Read the model definition and answer for the solid it produces. Units are mm, in the model's axes. Face numbers are marked on the shaded views. Give positions to 0.01 mm unless a question says otherwise; leave off trailing zeros. Write each loop counter-clockwise with the first axis right and the second up, starting at its lowest first coordinate (ties: lowest second). Pieces come first, ordered by that corner, then holes. Notation, with made-up numbers: M -16.5,-2 L -6.5,-2 A13 ccw -6.5,18 Z; hole C 5,-9 d1. An arc over 180 degrees is marked long. Write each question's results on one line, items separated by ' | '. Start each with the question number.
```python
from build123d import *

# Parameters (mm, degrees)
F0_R          = 76.2
F1_DEPTH      = 6.35
F3_R          = 38.1
F3_R_2        = 31.75
F4_DEPTH      = 6.35
F4_DEPTH_BACK = 6.35
F5_W          = 3.175
F5_H          = 3.175
F6_DEPTH      = 12.7


with BuildPart() as f1:
    # F0 (on Top) → F1 (new body)
    with BuildSketch(Plane.XY):
        Circle(F0_R)
        with BuildLine():
            Line((-41.613887, -47.963887), (-23.981943, -30.331943))
            Line((-23.981943, -30.331943), (-6.35, -63.181702))
            ThreePointArc((-6.35, -63.181702), (-25.160069, -58.302838), (-41.613887, -47.963887))
        make_face(mode=Mode.SUBTRACT)
        with BuildLine():
            ThreePointArc((-47.963887, -41.613887), (-58.302838, -25.160069), (-63.181702, -6.35))
            Line((-63.181702, -6.35), (-6.35, -6.35))
            Line((-6.35, -6.35), (-47.963887, -41.613887))
        make_face(mode=Mode.SUBTRACT)
        with BuildLine():
            Line((6.35, -63.181702), (6.35, -37.940851))
            Line((6.35, -37.940851), (41.613887, -47.963887))
            ThreePointArc((41.613887, -47.963887), (25.160069, -58.302838), (6.35, -63.181702))
        make_face(mode=Mode.SUBTRACT)
        with BuildLine():
            Line((47.963887, -41.613887), (6.35, -6.35))
            Line((6.35, -6.35), (63.181702, -6.35))
            ThreePointArc((63.181702, -6.35), (58.302838, -25.160069), (47.963887, -41.613887))
        make_face(mode=Mode.SUBTRACT)
        with BuildLine():
            Line((-6.35, 63.181702), (-5.498498, 19.546218))
            Line((-5.498498, 19.546218), (-8.109563, 21.600755))
            Line((-8.109563, 21.600755), (-6.35, 6.35))
            Line((-6.35, 6.35), (-63.181702, 6.35))
            ThreePointArc((-63.181702, 6.35), (-56.377813, 29.219723), (-41.613887, 47.963887))
            ThreePointArc((-41.613887, 47.963887), (-28.119246, 56.934682), (-12.793478, 62.197885))
            ThreePointArc((-12.793478, 62.197885), (-9.584371, 62.772525), (-6.35, 63.181702))
        make_face(mode=Mode.SUBTRACT)
        with BuildLine():
            Line((10.118387, 39.011938), (6.35, 37.940851))
            Line((6.35, 37.940851), (6.35, 63.181702))
            ThreePointArc((6.35, 63.181702), (9.584371, 62.772525), (12.793478, 62.197885))
            ThreePointArc((12.793478, 62.197885), (28.119246, 56.934682), (41.613887, 47.963887))
            ThreePointArc((41.613887, 47.963887), (56.377813, 29.219723), (63.181702, 6.35))
            Line((63.181702, 6.35), (6.35, 6.35))
            Line((6.35, 6.35), (10.118387, 39.011938))
        make_face(mode=Mode.SUBTRACT)
    extrude(amount=F1_DEPTH)

    # F3 (on offset) → F4 (join, two sides)
    with BuildSketch(Plane.XY.offset(3.175)) as f4_sk:
        Circle(F3_R)
        Circle(F3_R_2, mode=Mode.SUBTRACT)
    extrude(amount=F4_DEPTH)
    extrude(f4_sk.sketch, amount=-F4_DEPTH_BACK)

    # F5 (on Top) → F6 (cut, symmetric)
    with BuildSketch(Plane.XY):
        Rectangle(F5_W, F5_H)
    extrude(amount=F6_DEPTH, both=True, mode=Mode.SUBTRACT)


solid = f1.part
```
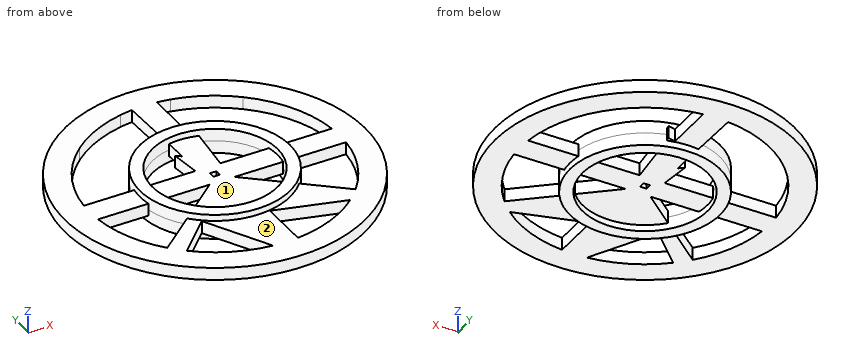
Item 1: Determine the mould class of the marked faces 1 and 2 for opening direction Y: +Y half, -Y half, draft (parallel to the pull), parting line (faces both ways), or undercut.
Item 2: Section B-B, the plane x = 55 is taken. Determine the outline of the cut face in (y, z).
Item 3: Section D-D, the plane y = -18 is taken. Give the number of separate pieces and of enclosed holes in the cut face, then the cut area to 3 significant figures.
Item 4: Straight lines are drawn through the part: line 1 (Y direction, x = 0, z = -0.5); line 2 (X direction, y = -49.5, z = 1.5); line 3 (X direction, y = -53, z = 4) (3 decimals). For each, find the intervals that lie inside material, in ascending order.
Item 5: Section C-C, the plane y = -60 is taken. Determine the outline of the cut face in (x, z), then the cut area to 3 significant figures.
Item 6: Given P1, Ø19, axis at x = 12.5, y = -13, coming from the +Z side; P2, Ø7, axis at y = 51.5, z = 2, coming from the +X side; P3, Ø1, axis at x = 0, z = 3, coming from the -Y side, each flat-ended and moving along its own axis, determine where each tip first touches the part or whether it passes through.
Item 7: Section A-A, the plane y = 12 is taken. Determine the outline of the cut face in (x, z) (3 decimals).
Worked out:
1) face 1: undercut | face 2: draft
2) outline: M -52.74,0 L -31.74,0 L -31.74,6.35 L -52.74,6.35 Z; M -6.35,0 L 6.35,0 L 6.35,6.35 L -6.35,6.35 Z; M 31.74,0 L 52.74,0 L 52.74,6.35 L 31.74,6.35 Z
3) separate pieces: 5 | enclosed holes: 0 | area: 611 mm²
4) line 1: y = -38.1 to -31.75, 31.75 to 38.1 | line 2: x = -57.93 to -39.77, -13.69 to 6.35, 39.77 to 57.93 | line 3: x = -54.749 to -34.975, -11.815 to 6.35, 34.975 to 54.749
5) outline: M -46.97,0 L -20.79,0 L -20.79,6.35 L -46.97,6.35 Z; M -8.06,0 L 6.35,0 L 6.35,6.35 L -8.06,6.35 Z; M 20.79,0 L 46.97,0 L 46.97,6.35 L 20.79,6.35 Z | area: 424 mm²
6) P1: stops at z = 6.35 | P2: stops at x = 59.18 | P3: stops at y = -76.2
7) outline: M -75.249,0 L -62.356,0 L -62.356,6.35 L -75.249,6.35 Z; M -36.161,-3.175 L -29.395,-3.175 L -29.395,9.525 L -36.161,9.525 Z; M -7.002,0 L 7.002,0 L 7.002,6.35 L -7.002,6.35 Z; M 29.395,-3.175 L 36.161,-3.175 L 36.161,9.525 L 29.395,9.525 Z; M 62.356,0 L 75.249,0 L 75.249,6.35 L 62.356,6.35 Z
